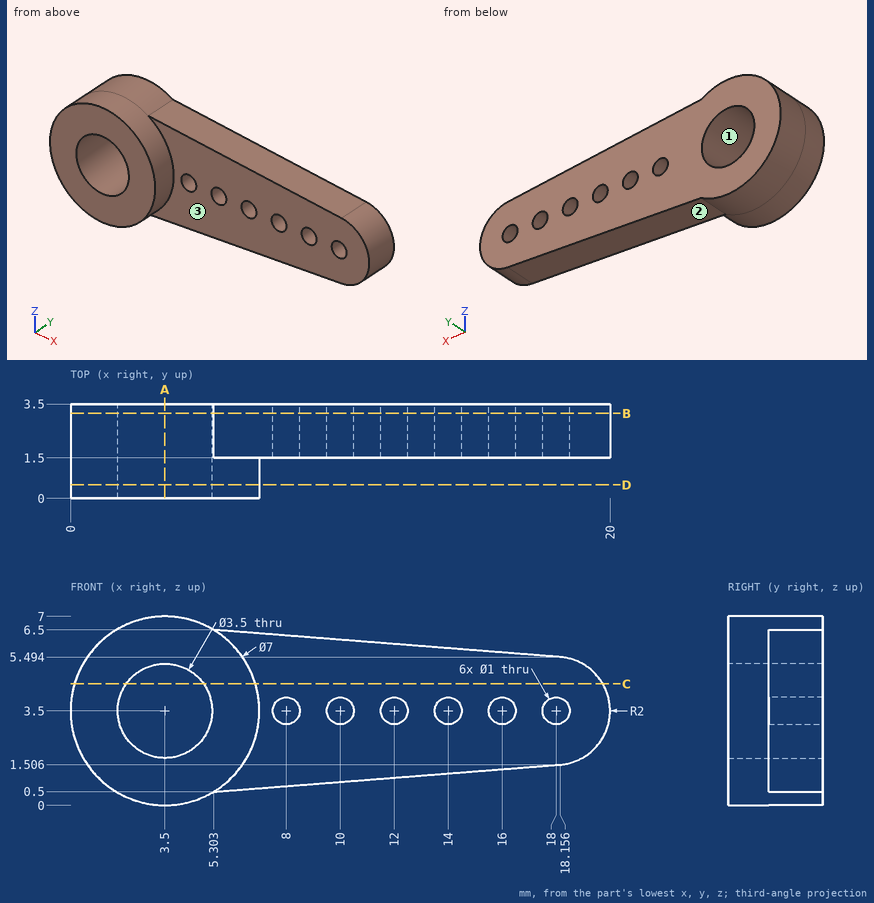
Geometry: see drawing. Coordinates: mm, zero at the bounding-box minimum. Give positions to 0.01 mm unless a question says otherwise; leave off trailing zeros. Loops run counter-clockwise (first coordinate to the right, second up) from the corner with the lowest first, then second, coordinate; pieces in that order, holes last. Notation, with made-up numbers: M -1,-8 L 11,-8 A34 cw 11,22 Z; hole C 80,43 d3. An arc over 180 degrees is marked long. Use one line per item in the form item = value.
1. Section query D-D, the plane y = 0.5. Return the cut outline in (x, z).
Numbers:
outline = C 3.5,3.5 d7; hole C 3.5,3.5 d3.5
2. Line query: L1, parallel to Y at x = 10.75, z = 4.25; L2, parallel to Z at x = 3.75, y = 1.25; L3, parallel to X at y = 1.4, z = 5. Output: solid intervals per line, ascending.
Numbers:
L1 = 1.5 to 3.5
L2 = 0.01 to 1.77, 5.23 to 6.99
L3 = 0.34 to 2.6, 4.4 to 6.66
3. Section query B-B, the plane y = 3.15. Return the cut outline in (x, z), and give its area (3 significant figures).
Numbers:
outline = M 5.3,0.5 L 18.16,1.51 A2 ccw 18.16,5.49 L 5.3,6.5 A3.5 ccw long Z; hole C 3.5,3.5 d3.5; hole C 8,3.5 d1; hole C 10,3.5 d1; hole C 12,3.5 d1; hole C 14,3.5 d1; hole C 16,3.5 d1; hole C 18,3.5 d1
area = 86.8 mm²
4. First-contact query: pin 1 (4 mm diameter, centred on x = 13, z = 5.5, fed in from -Y); pin 2 (2 mm diameter, centred on y = 2, z = 5, fed in from -X); pin 3 (1.5 mm diameter, centred on x = 11, y = 2, fed in from +Z); pin 4 (4 mm diameter, centred on x = 3.5, z = 3.5, fed in from +Y). Flat tips, straight axial feed; report the tip coordinate or a pass-through.
Numbers:
pin_1 = 1.5
pin_2 = 0.04
pin_3 = 6.11
pin_4 = 3.5
5. Section query C-C, the plane z = 4.5. Return the cut outline in (x, y).
Numbers:
outline = M 0.15,0 L 2.06,0 L 2.06,3.5 L 0.15,3.5 Z; M 4.94,0 L 6.85,0 L 6.85,1.5 L 19.73,1.5 L 19.73,3.5 L 4.94,3.5 Z
6. Section query A-A, the plane x = 3.5. Return the cut outline in (y, z).
Numbers:
outline = M 0,0 L 3.5,0 L 3.5,1.75 L 0,1.75 Z; M 0,5.25 L 3.5,5.25 L 3.5,7 L 0,7 Z
7. Pull-direction query (X, two-part tool) for the marked faces 1, 2 and 3; classes: released by +X, released by -X, zero draft, split by the parting line, or undercut.
Numbers:
face_1 = undercut
face_2 = released by +X
face_3 = zero draft
